from build123d import *

# Parameters (mm, degrees)
SKETCH1_R           = 5
BOSS_EXTRUDE1_DEPTH = 10
FILLET1_R           = 2.54
SCALE1_SCALE        = 0.66
FILLET2_R           = 1.27


with BuildPart() as part:
    # Sketch1 → Boss-Extrude1 (new body)
    with BuildSketch(Plane(origin=(0, 0, 0), x_dir=(1, 0, 0), z_dir=(0, 1, 0))):
        with BuildLine():
            Line((-37.807044038, -9.361111111), (33.524622629, -36.160986681))
            ThreePointArc((33.524622629, -36.160986681), (45.851500304, -31.531347991), (42.90340673, -18.698023718))
            Line((42.90340673, -18.698023718), (5.861740063, 8.101851852))
            ThreePointArc((5.861740063, 8.101851852), (3.080704585, 9.513635439), (0, 10))
            Line((0, 10), (-34.29, 10))
            ThreePointArc((-34.29, 10), (-44.128981429, 1.787300882), (-37.807044038, -9.361111111))
        make_face()
        with Locations((-34.29, 0)):
            Circle(SKETCH1_R, mode=Mode.SUBTRACT)
        Circle(SKETCH1_R, mode=Mode.SUBTRACT)
        with Locations((37.041666667, -26.79987557)):
            Circle(SKETCH1_R, mode=Mode.SUBTRACT)
        Polygon((-7.373318213, -14.24424589), (-27.557795825, -6.660776812), (-9.089196081, 1.165091942), align=None, mode=Mode.SUBTRACT)
        Polygon((10.448030186, -4.7063742), (5.617045705, -17.564724), (28.147439019, -26.029572301), align=None, mode=Mode.SUBTRACT)
    extrude(amount=BOSS_EXTRUDE1_DEPTH)

    # Fillet1
    fillet1_edges = [part.edges().sort_by_distance(p)[0] for p in [
        (45.851500304, 10, 31.531347991),
        (24.382573397, 10, 5.298085933),
        (3.080704585, 10, -9.513635439),
        (-17.145, 10, -10),
        (-44.128981429, 10, -1.787300882),
        (-17.145, 0, -10),
        (3.080704585, 0, -9.513635439),
        (24.382573397, 0, 5.298085933),
        (-2.141210705, 10, 22.761048896),
        (45.851500304, 0, 31.531347991),
        (-2.141210705, 0, 22.761048896),
        (-44.128981429, 0, -1.787300882),
    ]]
    fillet(fillet1_edges, radius=FILLET1_R)


with BuildPart() as part_1:
    # Scale1: scaled about (2.327239798, 5, 10.366216283)
    add(part.part.scale(SCALE1_SCALE).moved(Location((0.791261531, 1.7, 3.524513536))))

    # Fillet2
    fillet2_edges = [part_1.edges().sort_by_distance(p)[0] for p in [
        (-4.075128489, 5, 12.925715824),
        (-5.207607882, 5, 2.755552855),
        (-17.396883713, 5, 7.920626232),
        (19.368571284, 5, 20.704031255),
        (7.686961454, 5, 6.630720508),
        (4.498511697, 5, 15.117231376),
    ]]
    fillet(fillet2_edges, radius=FILLET2_R)


solid = part_1.part
Geometry: final body of the model. Coordinates: model frame, mm. A direction names the side the tool comes from. Round coordinates to 2 decimals unless told otherwise and drop trailing zeros. Loops run counter-clockwise (first coordinate to the right, second up) from the corner with the lowest first, then second, coordinate; pieces in that order, holes last. Notation, with made-up numbers: (-35, 7) - (3, 7) arc R21 ccw to (3, 28) - close; hole circle Ø11 at (13.25, 20). An arc over 180 degrees is marked (long way). Write each question's results on one line, items separated by ' | '. Start each with the question number.
1) Cut plane A-A on y = 7.75. Return loops of the section in (x, z), then the cut area to 3 significant figures.
2) Cut plane B-B on z = 1.5. Count the separate pieces of the cut face and the enclosed holes in it, then the cut area to 3 significant figures.
3) First-contact query: P1, Ø1.5, axis at y = 2.5, z = 10.5, coming from the +X side. Flat tip, straight axial feed; report the tip coordinate or a pass-through.
4) Cut plane C-C on y = 4.5. Return loops of the section in (x, z).
5) Line query: probe 1 along X at (y, z) = (6, 5); probe 2 along Z at (x, y) = (-19.5, 7.5); probe 3 along Z at (x, y) = (-19, 5). Output: solid intervals per line, ascending. Write a range as [from, to].
6) Access query for faces 1 (the face through (16.432, 7.796, 7.285)), 2 (the face through (10.223, 4.954, 17.268)). Directions: +Z, -Z, +X, -X, +Y, -Y. A direction counts if a zero-diameter tool reaches every point of the face in a straight line with its end or side. Return the directions, or none.
7) Mould query, pull axis X, two halves, no side actions, for faces 3 (the face through (7.878, 5.046, 7.876)), 4 (the face through (-28.31, 4.98, 2.22)), 5 (the face through (2, 1.7, 10)), 6 (the face through (-10.677, 4.954, 5.073)). Classes: released by +X, released by -X, zero draft, split by the parting line, or undercut.
Verdict:
1) outline: (-24.01, 9.3) arc R6.17 ccw to (-21.84, -2.64) - (0.79, -2.64) arc R6.17 ccw to (4.41, -1.47) - (28.85, 16.22) arc R6.17 ccw to (23.07, 26.98) - close; hole circle Ø6.6 at (-21.84, 3.52); hole (-14.47, 6.68) - (-6.78, 3.42) arc R1.27 ccw to (-5.02, 4.45) - (-4.3, 10.87) arc R1.27 ccw to (-6.01, 12.2) - (-14.42, 9.04) arc R1.27 ccw to start; hole circle Ø6.6 at (0.79, 3.52); hole (4.95, 13.93) - (6.92, 8.68) arc R1.27 ccw to (9.08, 8.31) - (16.31, 17.02) arc R1.27 ccw to (14.89, 19.02) - (5.69, 15.56) arc R1.27 ccw to start; hole circle Ø6.6 at (25.24, 21.21) | area: 725 mm2
2) separate pieces: 3 | enclosed holes: 0 | area: 175 mm2
3) P1: stops at x = 22.47
4) outline: (-24.16, 9.7) arc R6.6 ccw to (-21.84, -3.08) - (0.79, -3.08) arc R6.6 ccw to (4.66, -1.82) - (29.11, 15.87) arc R6.6 ccw to (22.92, 27.39) - close; hole circle Ø6.6 at (-21.84, 3.52); hole (-14.47, 6.68) - (-6.78, 3.42) arc R1.27 ccw to (-5.02, 4.45) - (-4.3, 10.87) arc R1.27 ccw to (-6.01, 12.2) - (-14.42, 9.04) arc R1.27 ccw to start; hole circle Ø6.6 at (0.79, 3.52); hole (4.95, 13.93) - (6.92, 8.68) arc R1.27 ccw to (9.08, 8.31) - (16.31, 17.02) arc R1.27 ccw to (14.89, 19.02) - (5.69, 15.56) arc R1.27 ccw to start; hole circle Ø6.6 at (25.24, 21.21)
5) probe 1: x = [-28.27, -24.79], [-18.89, -10.5], [-4.96, -2.16], [3.74, 14.09] | probe 2: z = [-2.83, 1.2], [5.85, 11.19] | probe 3: z = [-3.08, 1.84], [5.2, 11.64]
6) face 1: -Z, +X, +Y | face 2: +Y, -Y
7) face 3: undercut | face 4: released by -X | face 5: zero draft | face 6: undercut
